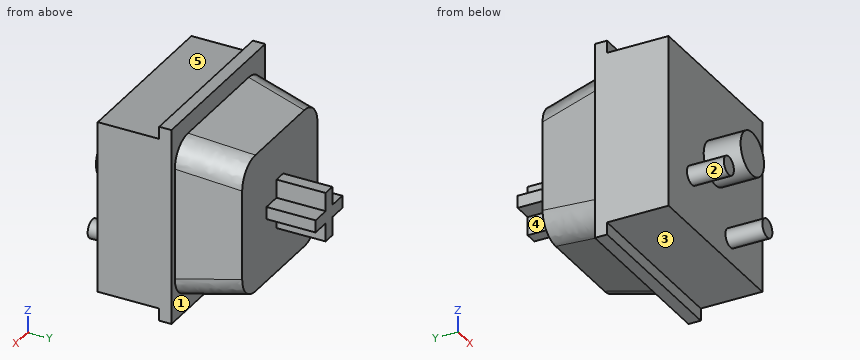
```python
from build123d import *

# Parameters (mm, degrees)
SKETCH1_W           = 14
SKETCH1_H           = 14
BOSS_EXTRUDE1_DEPTH = 5
SKETCH2_W           = 14
SKETCH2_H           = 16
BOSS_EXTRUDE2_DEPTH = 1
SKETCH3_W           = 13
SKETCH3_H           = 13
BOSS_EXTRUDE3_DEPTH = 5
BOSS_EXTRUDE3_TAPER = 10
BOSS_EXTRUDE4_DEPTH = 4
SKETCH5_R           = 1.75
BOSS_EXTRUDE5_DEPTH = 3
SKETCH6_R           = 0.75
BOSS_EXTRUDE6_DEPTH = 3
FILLET1_R           = 2


with BuildPart() as part:
    # Sketch1 → Boss-Extrude1 (new body)
    with BuildSketch(Plane(origin=(0, 0, 0), x_dir=(1, 0, 0), z_dir=(0, 1, 0))):
        Rectangle(SKETCH1_W, SKETCH1_H)
    extrude(amount=BOSS_EXTRUDE1_DEPTH)

    # Sketch2 → Boss-Extrude2 (add)
    with BuildSketch(Plane(origin=(0, 5, 0), x_dir=(1, 0, 0), z_dir=(0, 1, 0))):
        Rectangle(SKETCH2_W, SKETCH2_H)
    extrude(amount=BOSS_EXTRUDE2_DEPTH)

    # Sketch3 → Boss-Extrude3 (add)
    with BuildSketch(Plane(origin=(0, 6, 0), x_dir=(1, 0, 0), z_dir=(0, 1, 0))):
        Rectangle(SKETCH3_W, SKETCH3_H)
    extrude(amount=BOSS_EXTRUDE3_DEPTH, taper=BOSS_EXTRUDE3_TAPER)

    # Sketch4 → Boss-Extrude4 (add)
    with BuildSketch(Plane(origin=(0, 11, 0), x_dir=(1, 0, 0), z_dir=(0, 1, 0))):
        Polygon((0.5, -0.5), (2, -0.5), (2, 0.5), (0.5, 0.5), (0.5, 2), (-0.5, 2), (-0.5, 0.5), (-2, 0.5), (-2, -0.5), (-0.5, -0.5), (-0.5, -2), (0.5, -2), align=None)
    extrude(amount=BOSS_EXTRUDE4_DEPTH)

    # Sketch5 → Boss-Extrude5 (add)
    with BuildSketch(Plane.XZ):
        with Locations(Location((0, 0, 0), (0, 0, 270))):
            Circle(SKETCH5_R)
    extrude(amount=BOSS_EXTRUDE5_DEPTH)

    # Sketch6 → Boss-Extrude6 (add)
    with BuildSketch(Plane.XZ):
        with Locations(Location((2.25, -5, 0), (0, 0, 270))):
            Circle(SKETCH6_R)
        with Locations(Location((-3.5, -2.75, 0), (0, 0, 270))):
            Circle(SKETCH6_R)
    extrude(amount=BOSS_EXTRUDE6_DEPTH)

    # Fillet1
    fillet1_edges = [part.edges().sort_by_distance(p)[0] for p in [
        (6.059182548, 8.5, 6.059182548),
        (6.059182548, 8.5, -6.059182548),
        (-6.059182548, 8.5, -6.059182548),
        (-6.059182548, 8.5, 6.059182548),
    ]]
    fillet(fillet1_edges, radius=FILLET1_R)


solid = part.part
```
Verification items for the finished model (mm, model axes). Face numbers are marked on the shaded views. A direction names the side the tool comes from. Give positions to 0.01 mm unless a question says otherwise; leave off trailing zeros. Write each loop counter-clockwise with the first axis right and the second up, starting at its lowest first coordinate (ties: lowest second). Pieces come first, ordered by that corner, then holes. Notation, with made-up numbers: (-40, 4.5) - (-20, 4.5) arc R23 cw to (-20, 31.5) - close; hole circle Ø8 at (-6, 65.5). An arc over 180 degrees is marked (long way). Put each result on its own line as item: value.
Q1. Section check C-C on y = 0.5. Record the cut outline in (x, z), and give its area (3 significant figures).
Result:
outline: (-7, -7) - (7, -7) - (7, 7) - (-7, 7) - close
area: 196 mm2
Q2. Scan lines: probe 1 along Y at (x, z) = (2.75, -5.25); probe 2 along Y at (x, z) = (5.5, -1.5); probe 3 along Z at (x, y) = (6, 2.75). Record each from-to range of solid material in increasing order. Write a range as from..to.
Result:
probe 1: -3..11
probe 2: 0..11
probe 3: -7..7
Q3. Depth check by flat-ended pin: P1, Ø0.8, axis at y = 13.5, z = 0, coming from the +X side; P2, Ø1.5, axis at x = -2.5, z = 2.5, coming from the +Y side; P3, Ø1.6, axis at x = 1, y = 13, coming from the -Z side. Enter the tip coordinate at first touch or a pass-through.
Result:
P1: x = 2
P2: y = 11
P3: z = -2
Q4. Section check A-A on y = 13. Record the cut outline in (x, z).
Result:
outline: (-2, -0.5) - (-0.5, -0.5) - (-0.5, -2) - (0.5, -2) - (0.5, -0.5) - (2, -0.5) - (2, 0.5) - (0.5, 0.5) - (0.5, 2) - (-0.5, 2) - (-0.5, 0.5) - (-2, 0.5) - close
Q5. Section check B-B on z = 7.25. Record the cut outline in (x, y), and give its area (3 significant figures).
Result:
outline: (-7, 5) - (7, 5) - (7, 6) - (-7, 6) - close
area: 14.0 mm2
Q6. Set-up check for the marked faces 1, 2, 3, 4 and 5: record each of +Z, -Z, +X, -X, +Y, -Y from which the full face is reachable in a straight line by a thin tool's end or side.
Result:
face 1: +Y
face 2: -Y
face 3: -Z, +X, -X, -Y
face 4: -Z, -X, +Y
face 5: +Z, +X, -X, -Y
